from build123d import *

# Parameters (mm, degrees)
RESSALTO_EXTRUS_O1_DEPTH = 2
CORTE_EXTRUS_O1_REACH    = 4
ESBO_O2_R                = 2.1
CORTE_EXTRUS_O2_DEPTH    = 10


with BuildPart() as part:
    # Esboço1 → Ressalto-extrusão1 (new body)
    with BuildSketch(Plane.XY):
        Polygon((56.463679973, 135.159747673), (-55.864365487, 135.159747673), (-94.700342757, 88.87683224), (-94.700342757, 23.490318666), (-49.700342757, -30.138593001), (-49.700342757, -133.732537696), (-48.380219867, -134.840252327), (48.979534352, -134.840252327), (50.299657243, -133.732537696), (50.299657243, -30.138593001), (95.299657243, 23.490318666), (95.299657243, 88.87683224), align=None)
    extrude(amount=RESSALTO_EXTRUS_O1_DEPTH)

    # Esboço2 → Corte-extrusão1 (cut, up to next)
    with BuildSketch(Plane.XY.offset(2), mode=Mode.PRIVATE) as corte_extrus_o1_sk1:
        with Locations((-71.672714117, 109.298736063)):
            Circle(ESBO_O2_R)
    corte_extrus_o1_tool1 = extrude(corte_extrus_o1_sk1.sketch, amount=-CORTE_EXTRUS_O1_REACH, mode=Mode.PRIVATE) & part.part
    add(corte_extrus_o1_tool1.solids().sort_by_distance((-71.672714, 109.298736, 2))[0], mode=Mode.SUBTRACT)
    # Esboço2 → Corte-extrusão1 (cut, up to next)
    with BuildSketch(Plane.XY.offset(2), mode=Mode.PRIVATE) as corte_extrus_o1_sk2:
        with Locations((-45.200342757, -129.610252327)):
            Circle(ESBO_O2_R)
    corte_extrus_o1_tool2 = extrude(corte_extrus_o1_sk2.sketch, amount=-CORTE_EXTRUS_O1_REACH, mode=Mode.PRIVATE) & part.part
    add(corte_extrus_o1_tool2.solids().sort_by_distance((-45.200343, -129.610252, 2))[0], mode=Mode.SUBTRACT)
    # Esboço2 → Corte-extrusão1 (cut, up to next)
    with BuildSketch(Plane.XY.offset(2), mode=Mode.PRIVATE) as corte_extrus_o1_sk3:
        with Locations((45.799657243, -129.610252327)):
            Circle(ESBO_O2_R)
    corte_extrus_o1_tool3 = extrude(corte_extrus_o1_sk3.sketch, amount=-CORTE_EXTRUS_O1_REACH, mode=Mode.PRIVATE) & part.part
    add(corte_extrus_o1_tool3.solids().sort_by_distance((45.799657, -129.610252, 2))[0], mode=Mode.SUBTRACT)
    # Esboço2 → Corte-extrusão1 (cut, up to next)
    with BuildSketch(Plane.XY.offset(2), mode=Mode.PRIVATE) as corte_extrus_o1_sk4:
        with Locations((72.272028603, 109.298736063)):
            Circle(ESBO_O2_R)
    corte_extrus_o1_tool4 = extrude(corte_extrus_o1_sk4.sketch, amount=-CORTE_EXTRUS_O1_REACH, mode=Mode.PRIVATE) & part.part
    add(corte_extrus_o1_tool4.solids().sort_by_distance((72.272029, 109.298736, 2))[0], mode=Mode.SUBTRACT)
    # Esboço2 → Corte-extrusão1 (cut, up to next)
    with BuildSketch(Plane.XY.offset(2), mode=Mode.PRIVATE) as corte_extrus_o1_sk5:
        with Locations((-68.753142763, -0.431592924)):
            Circle(ESBO_O2_R)
    corte_extrus_o1_tool5 = extrude(corte_extrus_o1_sk5.sketch, amount=-CORTE_EXTRUS_O1_REACH, mode=Mode.PRIVATE) & part.part
    add(corte_extrus_o1_tool5.solids().sort_by_distance((-68.753143, -0.431593, 2))[0], mode=Mode.SUBTRACT)
    # Esboço2 → Corte-extrusão1 (cut, up to next)
    with BuildSketch(Plane.XY.offset(2), mode=Mode.PRIVATE) as corte_extrus_o1_sk6:
        with Locations((69.352457249, -0.431592924)):
            Circle(ESBO_O2_R)
    corte_extrus_o1_tool6 = extrude(corte_extrus_o1_sk6.sketch, amount=-CORTE_EXTRUS_O1_REACH, mode=Mode.PRIVATE) & part.part
    add(corte_extrus_o1_tool6.solids().sort_by_distance((69.352457, -0.431593, 2))[0], mode=Mode.SUBTRACT)

    # Esboço3 → Corte-extrusão2 (cut)
    with BuildSketch(Plane.XY.offset(2)):
        Polygon((-53.532827197, 130.159747673), (-64.879577854, 116.637216813), (-64.263293687, 109.593056549), (-70.675930858, 101.950773162), (-77.720091122, 101.334488995), (-89.700342757, 87.056981069), (-89.700342757, 25.310169837), (-74.789956765, 7.540663764), (-67.745796501, 6.924379597), (-61.334000151, -0.716901738), (-61.950284318, -7.761062002), (-44.700342757, -28.318741829), (-44.700342757, -117.173246706), (-31.407709232, -128.327090595), (32.007023717, -128.327090595), (45.299657243, -117.173246706), (45.299657243, -28.318741829), (62.549598803, -7.761062002), (61.933314636, -0.716901738), (68.345110987, 6.924379597), (75.389271251, 7.540663764), (90.299657243, 25.310169837), (90.299657243, 87.056981069), (78.319405608, 101.334488995), (71.275245343, 101.950773162), (64.862608173, 109.593056549), (65.47889234, 116.637216813), (54.132141682, 130.159747673), align=None)
    extrude(amount=-CORTE_EXTRUS_O2_DEPTH, mode=Mode.SUBTRACT)


solid = part.part
Verification items for the finished model (mm, model axes). A direction names the side the tool comes from. Coordinates: 2 decimals unless noted, no trailing zeros. Order: outer loops, then holes, each group sorted by start corner. A loop starts at its lowest first (then second) coordinate and runs counter-clockwise, first axis right, second up. Notation, with made-up numbers: M 39,33 L 56,33 A11 cw 56,40 Z; hole C -8,-33 d4. An arc over 180 degrees is marked long. Return JSON: item names as keys, results as strings.
1) Cross-section at B-B, the plane x = -22. Record the boundary of the cut face in (y, z), and give its area (3 significant figures).
Answer list:
{"outline": "M -134.84,0 L -128.33,0 L -128.33,2 L -134.84,2 Z; M 130.16,0 L 135.16,0 L 135.16,2 L 130.16,2 Z", "area": "23.0 mm2"}
2) Cross-section at C-C, the plane z = 1.45. Count the separate pieces of the cut face and the enclosed holes in it, and give its area (3 significant figures).
Answer list:
{"separate pieces": "1", "enclosed holes": "7", "area": "4,470 mm2"}
3) Access from +Z, -Z, +X, -X, +Y, -Y to the whole of each face (thin tool, end or side, straight path). Record for faces 5 (the flat face through (72.485, -3.7, 0.986)), 6 (the flat face through (53.804, -18.184, 1.014)).
Answer list:
{"face 5": "+Z, -Z, +X, -Y", "face 6": "+Z, -Z"}
4) Cross-section at A-A, the plane y = -107.5. Record the boundary of the cut face in (x, z), and give its area (3 significant figures).
Answer list:
{"outline": "M -49.7,0 L -44.7,0 L -44.7,2 L -49.7,2 Z; M 45.3,0 L 50.3,0 L 50.3,2 L 45.3,2 Z", "area": "20.0 mm2"}
5) Gauge pin test, flat ends, axial feed: pin 1 (4 mm diameter, centred on x = -68.75, y = -0.43, fed in from +Z); pin 2 (5.5 mm diameter, centred on x = 72.27, y = 109.3, fed in from -Z). Record the tip position at first contact, or that the pin passes through.
Answer list:
{"pin 1": "through", "pin 2": "z = 0"}
6) Release check for a two-part mould opening along X. For faces 1 (the flat face through (-64.585, 3.157, 1.014)), 2 (the flat face through (-49, -29, 0)), 3 (the flat face through (76.154, 111.694, 0.986)), 4 (the flat face through (-72.515, -2.949, 0.986)) record: +X half, -X half, draft (parallel to the pull), parting line (faces both ways), or undercut.
Answer list:
{"face 1": "undercut", "face 2": "draft", "face 3": "+X half", "face 4": "-X half"}
7) Thickness scan on L1, parallel to X at y = -47.5, z = 0.8; L2, parallel to Y at x = 17.5, z = 1.8; L3, parallel to Y at x = -71.5, z = 0.15. Record the ranges inside material, lowest first. Write a range as [from, to].
Answer list:
{"L1": "[-49.7, -44.7], [45.3, 50.3]", "L2": "[-134.84, -128.33], [130.16, 135.16]", "L3": "[-4.16, 7.25], [101.88, 107.21], [111.39, 116.53]"}
